Geometry: final body of the model. Coordinates: model frame, mm. A direction names the side the tool comes from. Round coordinates to 2 decimals unless told otherwise and drop trailing zeros. Write each loop counter-clockwise with the first axis right and the second up, starting at its lowest first coordinate (ties: lowest second). Pieces come first, ordered by that corner, then holes. Notation, with made-up numbers: (61, 89.25) - (68, 89.25) arc R19 cw to (68, 124.25) - close; hole circle Ø7 at (-20.5, 9). An arc over 180 degrees is marked (long way). Write each question's results on one line, items separated by ' | '.
Autodesk Inventor part; units mm, degrees
ref_plane "XZ Plane" through (0, 0, 0) normal (0, 1, 0) x (-1, 0, 0)
ref_plane "XY Plane" through (0, 0, 0) normal (0, 0, 1) x (1, 0, 0)
sketch "Sketch1" plane through (0, 0, 0) normal (0, 0, 1) x (1, 0, 0)
  arc A0 (0, 15.3683) -> (-19.6378, -9.7289) centre (-2.7904, -2.6799) ccw
  arc A1 (-5.842, 16.6129) -> (-21.0429, -9.6347) centre (-2.7904, -2.6799) ccw
  line L0 (0, 51.5125) -> (-5.842, 51.5125)
  line L1 (-5.842, 51.5125) -> (-5.842, 16.6129)
  line L2 (0, 15.3683) -> (0, 51.5125)
  arc A2 (0, 15.3683) -> (-17.0727, -14.0614) centre (-2.7904, -2.6799) ccw
  arc A3 (0, 16.6524) -> (-18.6644, -14.0614) centre (-2.7904, -2.6799) ccw
  line L3 (-18.6644, -14.0614) -> (-17.0727, -14.0614)
  dimension "d3" = 1.27
  dimension "d5" = 34.8996
  dimension "d6" = 18.2626
  dimension "d7" = 5.842
  dimension "d9" = 36.1442
revolve "Revolution1" add sketch "Sketch1" angle 360 about axis through (0, 15.3683, 0) along (0, 1, 0)
sketch "Sketch4" plane through (0, 51.5125, 0) normal (0, 1, 0) x (1, 0, 0)
  circle A0 centre (0, 0) radius 5.842
  circle A1 centre (0, 0) radius 2.9972
  point P0 (0, 0)
  dimension "d21" = 5.9944
extrude "Cut1" cut sketch "Sketch4" against normal blind 3.048 contours A0 | A1
sketch "Sketch5" plane through (0, 0, 0) normal (1, 0, 0) x (0, 1, 0)
  line L0 (3.3342, -12.2505) -> (3.3342, 12.2505)
  circle A0 centre (3.3342, 0) radius 7.99
  point P0 (0, 0)
extrude "Extrusion3" cut sketch "Sketch5" along normal mid plane 25.4
sketch "Sketch6" plane through (0, 48.4645, 0) normal (0, 1, 0) x (1, 0, 0)
  circle A0 centre (0, 0) radius 2.9972
  point P0 (0, 0)
  dimension "d22" = 5.9944
extrude "Extrusion4" cut sketch "Sketch6" against normal blind 12.7
sketch "Sketch7" plane through (-12.7, 0, 0) normal (1, 0, 0) x (0, 0, -1)
  circle A0 centre (0, 6.8594) radius 3.3582
  point P0 (0, 0)
extrude "Extrusion5" [suppressed]
sketch "Sketch8" plane through (-12.7, 0, 0) normal (1, 0, 0) x (0, 0, -1)
  circle A0 centre (0.7643, 6.3089) radius 4.4927
  point P0 (0, 0)
extrude "Extrusion6" [suppressed]
sketch "Sketch9" plane through (12.7, 0, 0) normal (-1, 0, 0) x (0, 0, 1)
  circle A0 centre (0, 6.8376) radius 3.6987
  point P0 (0, 0)
extrude "Extrusion7" [suppressed]
fillet "Fillet1" radius 2.54 1 edges at (5.842, 16.6129, 0)
sketch "Sketch10" plane through (0, 0, 0) normal (1, 0, 0) x (0, 1, 0)
  line L0 (-14.0614, -17.0727) -> (-14.0614, 17.0727)
  circle A0 centre (-14.0614, 0) radius 11.9423
  point P0 (0, 0)
extrude "Extrusion8" cut sketch "Sketch10" against normal blind 25.4
sketch "Sketch11" plane through (0, 0, 0) normal (1, 0, 0) x (0, 1, 0)
  line L0 (-14.0614, -17.0727) -> (-14.0614, 17.0727)
  circle A0 centre (-14.0614, 0) radius 11.938
  point P0 (0, 0)
  point P1 (-14.0614, 11.9423)
  point P2 (-14.0614, -11.9423)
  dimension "d34" = 23.876
extrude "Extrusion9" cut sketch "Sketch11" along normal blind 25.4
equation "\"d17\" = Thickness"
equation "\"BendRadius\" = Thickness"
equation "\"BendReliefWidth\" = Thickness"
equation "\"BendReliefDepth\" = 0.5 * Thickness"
equation "\"CornerReliefSize\" = 4 * Thickness"
equation "\"MinimumRemnant\" = 2 * Thickness"
equation "\"TransitionRadius\" = BendRadius"
equation "\"JacobiRadiusSize\" = Thickness"
equation "\"GapSize\" = Thickness"
properties part number "mcdave caster"
Q1. Access query for faces 4 (the cylindrical face through (-21.35, -2.12, -0.09)), 5 (the flat face through (0, 35.764, 0)). Directions: +Z, -Z, +X, -X, +Y, -Y. A direction counts if a zero-diameter tool reaches every point of the face in a straight line with its end or side. Return the directions, or none.
Answer block:
face 4: +X, -X, -Y | face 5: +Y
Q2. Section query A-A, the plane y = 37. Return loops of the section in (x, z), plus the area to 3 significant figures.
Answer block:
outline: circle Ø11.68 at (0, 0); hole circle Ø5.99 at (0, 0) | area: 79.0 mm2
Q3. Pin query (flat end, axial travel): pin 1 (5 mm diameter, centred on x = 0, z = 0, fed in from +Y); pin 2 (2 mm diameter, centred on y = 6, z = -15, fed in from -X); pin 3 (5 mm diameter, centred on x = 13, y = 13.5, fed in from +Z). Return the tip coordinate at first contact, or that it passes through.
Answer block:
pin 1: y = 35.76 | pin 2: x = -14.89 | pin 3: z = 11.45
Q4. Mould query, pull axis Z, two halves, no side actions, for faces 1 (the cylindrical face through (1.266, 33.36, 5.703)), 2 (the flat face through (0, -14.061, -18)), 3 (the cylindrical face through (21.357, -2.124, 0.088)). Classes: pulls with the +Z half, pulls with the -Z half, needs draft (parallel to the pull), parting line crosses it, or undercut.
Answer block:
face 1: parting line crosses it | face 2: needs draft | face 3: undercut
Q5. Ray query, line 1 along Z through (x, y) = (13, 5); line 2 along X through (y, z) = (40, 0). Return the intervals inside material, ascending.
Answer block:
line 1: -16.17 to -14.35, 14.35 to 16.17 | line 2: -5.84 to -3, 3 to 5.84
Q6. Section query B-B, the plane y = 29.5. Return loops of the section in (x, z).
Answer block:
outline: circle Ø11.68 at (0, 0)
